from build123d import *

# Parameters (mm, degrees)
F1_DEPTH = 361.95
F2_R     = 117.475
F3_DEPTH = 25.4


with BuildPart() as f1:
    # F0 (on Right) → F1 (new body)
    with BuildSketch(Plane.YZ):
        Polygon((0, 344.4875), (0, 0), (295.275, 0), (217.4875, 344.4875), align=None)
    extrude(amount=F1_DEPTH)

    # F2 (on face) → F3 (cut)
    with BuildSketch(Plane.XZ):
        with Locations((180.975, 172.24375)):
            Circle(F2_R)
    extrude(amount=-F3_DEPTH, mode=Mode.SUBTRACT)


solid = f1.part
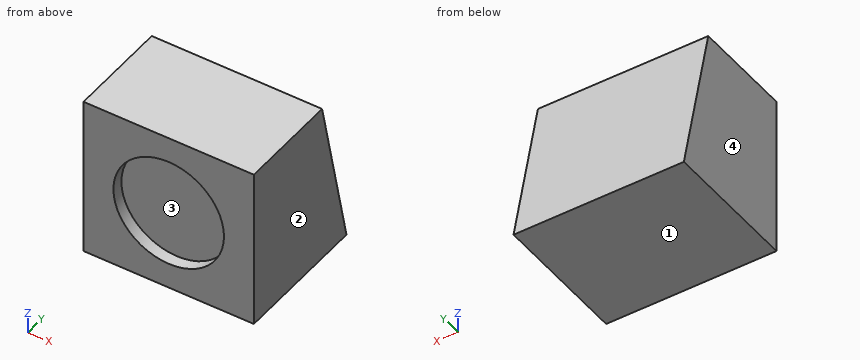
CAD build for the part. Positions are in the model's coordinates, mm. Face numbers are marked on the shaded views. Coordinates: 2 decimals unless noted, no trailing zeros. Loops run counter-clockwise (first coordinate to the right, second up) from the corner with the lowest first, then second, coordinate; pieces in that order, holes last. Notation, with made-up numbers: (15, 21) - (30, 21) arc R26 ccw to (30, 50) - close; hole circle Ø8 at (-23.75, -28.5). An arc over 180 degrees is marked (long way). Use one line per item in the form item = value. Start each with the question number.
1) Drill centre lines: L1, parallel to Y at x = 51.5, z = 70; L2, parallel to Y at x = 79, z = 81. Where is each one in solid material? Low to high. Write a range as from..to.
2) Two-plate mould, pull along X, no slides. Class the marked faces 1, 2, 3 and 4: +X half, -X half, draft (parallel to the pull), parting line (faces both ways), or undercut.
3) Band-saw the part on B-B (x = 129). Give the cut face in (y, z) (1 decimal).
4) Flat gauge pins, fed straight in: pin 1 (10 mm diameter, centred on x = 130, z = 212.5, fed in from -Y); pin 2 (12 mm diameter, centred on x = 76, z = 178.5, fed in from +Y); pin 3 (8 mm diameter, centred on x = 105, z = 108, fed in from +Y). Where does each tip first touch, or does it go through?
5) Band-saw the part on C-C (y = 262.5). Give the cut face in (x, z).
6) Band-saw the part on D-D (z = 44). Give the cut face in (x, y), and give its area (3 significant figures).
7) Band-saw the part on A-A (z = 196). Give the cut face in (x, y), and give its area (3 significant figures).
Check values:
q1.L1 = 0..279.47
q1.L2 = 0..276.98
q2.face_1 = draft
q2.face_2 = +X half
q2.face_3 = undercut
q2.face_4 = -X half
q3.outline = (0, 0) - (295.3, 0) - (217.5, 344.5) - (0, 344.5) - (0, 277.6) - (25.4, 277.6) - (25.4, 66.9) - (0, 66.9) - close
q4.pin_1 = 25.4
q4.pin_2 = 256.32
q4.pin_3 = 271.79
q5.outline = (0, 0) - (361.95, 0) - (361.95, 145.15) - (0, 145.15) - close
q6.outline = (0, 0) - (361.95, 0) - (361.95, 285.34) - (0, 285.34) - close
q6.area = 103,000 mm2
q7.outline = (0, 0) - (65.93, 0) - (65.93, 25.4) - (296.02, 25.4) - (296.02, 0) - (361.95, 0) - (361.95, 251.02) - (0, 251.02) - close
q7.area = 85,000 mm2
